from build123d import *

# Parameters (mm, degrees)
F0_W     = 19.05
F0_H     = 7.1882
F1_DEPTH = 2.54


with BuildPart() as f1:
    # F0 (on Top) → F1 (new body)
    with BuildSketch(Plane.XY):
        Polygon((-16.8275, -22.445938), (-9.525, -22.445938), (9.525, -22.445938), (16.8275, -22.445938), (16.8275, -4.234138), (-16.8275, -4.234138), align=None)
        with Locations((0, -26.040038)):
            Rectangle(F0_W, F0_H)
        with Locations((0, -33.228238)):
            Rectangle(F0_W, F0_H)
        Polygon((-9.525, -36.822338), (-16.8275, -36.822338), (-16.8275, -55.034138), (16.8275, -55.034138), (16.8275, -36.822338), (9.525, -36.822338), align=None)
    extrude(amount=-F1_DEPTH)


solid = f1.part
CAD build for the part. Positions are in the model's coordinates, mm. A direction names the side the tool comes from. Give positions to 0.01 mm unless a question says otherwise; leave off trailing zeros. Order: outer loops, then holes, each group sorted by start corner. A loop starts at its lowest first (then second) coordinate and runs counter-clockwise, first axis right, second up. Notation, with made-up numbers: (-40, 50) - (-29, 50) arc R20 cw to (-29, 87) - close; hole circle Ø1 at (-27.5, 61.5). An arc over 180 degrees is marked (long way). Answer in a Markdown table with one row per item.
1. Pull direction Y, two halves, no side cores. Call faces 1 (the flat face through (0, -55.034, -1)), 2 (the flat face through (9.525, -30, -1)), 3 (the flat face through (0, -29, -2.54)), 4 (the flat face through (0, -4.234, -1)): pulls with the +Y half, pulls with the -Y half, needs draft (parallel to the pull), parting line crosses it, or undercut.
Data:
| item | result |
|---|---|
| face 1 | pulls with the -Y half |
| face 2 | undercut |
| face 3 | needs draft |
| face 4 | pulls with the +Y half |
2. Saw through at A-A, the plane x = -12. Give the cut face in (y, z), plus the area to 3 significant figures.
Data:
| item | result |
|---|---|
| outline | (-55.03, -2.54) - (-36.82, -2.54) - (-36.82, 0) - (-55.03, 0) - close; (-22.45, -2.54) - (-4.23, -2.54) - (-4.23, 0) - (-22.45, 0) - close |
| area | 92.5 mm² |
3. Tool access for faces 5 (the flat face through (13, -22.446, -1)), 6 (the flat face through (0, -29, 0)), 7 (the flat face through (-9.525, -30, -1)): list every direction of +Z, -Z, +X, -X, +Y, -Y with a clear straight run to the whole face (end or side of a thin tool).
Data:
| item | result |
|---|---|
| face 5 | +Z, -Z, +X |
| face 6 | +Z, +X, -X, +Y, -Y |
| face 7 | +Z, -Z, -X |
4. Probe probe 1 along Y at (x, z) = (12.5, -0.75); probe 2 along X at (y, z) = (-28, -0.25) (3 decimals). List the from-to ranges inside material, lowest first. Write a range as [from, to].
Data:
| item | result |
|---|---|
| probe 1 | y = [-55.03, -36.82], [-22.45, -4.23] |
| probe 2 | x = [-9.525, 9.525] |
5. Saw through at B-B, the plane z = -1.6. Give the cut face in (x, y) (1 decimal), plus the area to 3 significant figures.
Data:
| item | result |
|---|---|
| outline | (-16.8, -55) - (16.8, -55) - (16.8, -36.8) - (9.5, -36.8) - (9.5, -22.4) - (16.8, -22.4) - (16.8, -4.2) - (-16.8, -4.2) - (-16.8, -22.4) - (-9.5, -22.4) - (-9.5, -36.8) - (-16.8, -36.8) - close |
| area | 1,500 mm² |
6. Flat gauge pin, fed straight in: pin 1 (1.3 mm diameter, centred on y = -32.5, z = -1.5, fed in from +X) (3 decimals). Where does the tip first touch, or does it go through?
Data:
| item | result |
|---|---|
| pin 1 | stops at x = 9.525 |
7. Saw through at C-C, the plane y = -28.5. Give the cut face in (x, z) (3 decimals).
Data:
| item | result |
|---|---|
| outline | (-9.525, -2.54) - (9.525, -2.54) - (9.525, 0) - (-9.525, 0) - close |
